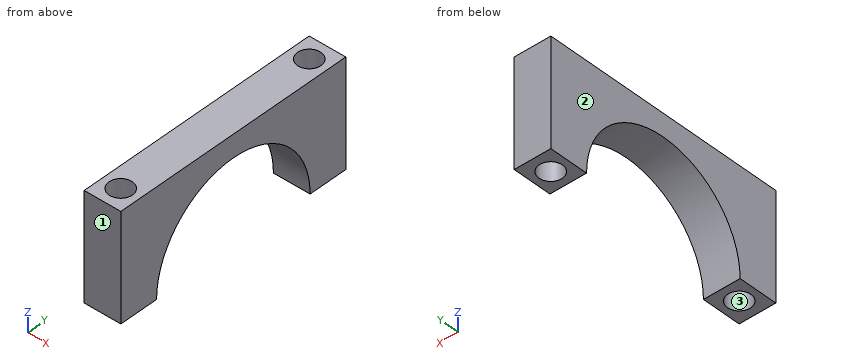
Autodesk Inventor part; units mm, degrees
ref_plane "YZ Plane" through (0, 0, 0) normal (1, 0, 0) x (0, 1, 0)
ref_plane "XZ Plane" through (0, 0, 0) normal (0, 1, 0) x (-1, 0, 0)
ref_plane "XY Plane" through (0, 0, 0) normal (0, 0, 1) x (1, 0, 0)
sketch "Sketch1" plane through (0, 0, 0) normal (0, 0, 1) x (1, 0, 0)
  line L0 (0, 0) -> (5.5, 0)
  line L1 (5.5, 0) -> (5.5, 37)
  line L2 (5.5, 37) -> (0, 37)
  line L3 (0, 37) -> (0, 0)
  point P0 (2.75, 34)
  point P1 (2.75, 3)
  dimension "d7" = 5.5
  dimension "d8" = 37
  dimension "d9" = 31
  dimension "d10" = 3
  dimension "d11" = 2.75
extrude "Extrusion4" add sketch "Sketch1" along normal blind 16
sketch "Sketch6" plane through (0, 0, 0) normal (0, 0, 1) x (1, 0, 0)
  line L0 (0, 0) -> (5.5, 0)
  line L1 (5.5, 0) -> (5.5, 37)
  line L2 (5.5, 37) -> (0, 37)
  line L3 (0, 37) -> (0, 0)
  point P0 (2.75, 34)
  point P1 (2.75, 3)
  dimension "d45" = 5.5
  dimension "d46" = 37
  dimension "d47" = 31
  dimension "d48" = 3
  dimension "d49" = 2.75
hole "Hole3" at (2.75, 34, 0) at (2.75, 3, 0) direction (0, 0, 1) diameter 3.5 end through all
sketch "Sketch7" plane through (5.5, 0, 0) normal (1, 0, 0) x (0, 0, -1)
  line L0 (0, 0) -> (0, 37)
  arc A0 (0, 31.125) -> (0, 5.875) centre (0, 18.5) ccw
  line L1 (0, 31.125) -> (0, 5.875)
  dimension "d59" = 25.25
extrude "Extrusion5" cut sketch "Sketch7" against normal blind 5.5
properties part number "SujetadorColaVTOL"
The listing builds one solid part. Answer for the finished solid, in the listing's coordinates (mm). Face numbers are marked on the shaded views. Give positions to 0.01 mm unless a question says otherwise; leave off trailing zeros. Order: outer loops, then holes, each group sorted by start corner. A loop starts at its lowest first (then second) coordinate and runs counter-clockwise, first axis right, second up. Notation, with made-up numbers: (15.5, 46.25) - (73.5, 46.25) arc R5 ccw to (73.5, 50.25) - close; hole circle Ø7 at (14, 68). An arc over 180 degrees is marked (long way). Answer as CSV lines item,"result".
Q1. A cutting plane is placed at D-D, the plane z = 2.25. Determine the outline of the cut face in (x, y), and give its area (3 significant figures).
Answer key:
outline,"(0, 0) - (5.5, 0) - (5.5, 6.08) - (0, 6.08) - close; (0, 30.92) - (5.5, 30.92) - (5.5, 37) - (0, 37) - close; hole circle Ø3.5 at (2.75, 3); hole circle Ø3.5 at (2.75, 34)"
area,"47.6 mm^2"
Q2. A cutting plane is placed at C-C, the plane x = 1.35. Determine the outline of the cut face in (y, z) (3 decimals).
Answer key:
outline,"(0, 0) - (1.95, 0) - (1.95, 16) - (0, 16) - close; (4.05, 0) - (5.875, 0) arc R12.625 cw to (31.125, 0) - (32.95, 0) - (32.95, 16) - (4.05, 16) - close; (35.05, 0) - (37, 0) - (37, 16) - (35.05, 16) - close"
Q3. A cutting plane is placed at B-B, the plane z = 4. Determine the outline of the cut face in (x, y).
Answer key:
outline,"(0, 0) - (5.5, 0) - (5.5, 6.53) - (0, 6.53) - close; (0, 30.47) - (5.5, 30.47) - (5.5, 37) - (0, 37) - close; hole circle Ø3.5 at (2.75, 3); hole circle Ø3.5 at (2.75, 34)"
Q4. Determine the mould class of the marked faces 1, 2 and 3 for opening direction Y: pulls with the +Y half, pulls with the -Y half, needs draft (parallel to the pull), parting line crosses it, or undercut.
Answer key:
face 1,"pulls with the -Y half"
face 2,"needs draft"
face 3,"undercut"
Q5. A cutting plane is placed at A-A, the plane y = 3. Determine the outline of the cut face in (x, z).
Answer key:
outline,"(0, 0) - (1, 0) - (1, 16) - (0, 16) - close; (4.5, 0) - (5.5, 0) - (5.5, 16) - (4.5, 16) - close"
Q6. Straight lines are drawn through the part: L1, parallel to Y at x = 2.75, z = 6; L2, parallel to Y at x = 4.3, z = 7.25; L3, parallel to X at y = 3, z = 4.75. For each, find the intervals that lie inside material, in ascending order.
Answer key:
L1,"y = 0 to 1.25, 4.75 to 7.39, 29.61 to 32.25, 35.75 to 37"
L2,"y = 0 to 2.19, 3.81 to 8.16, 28.84 to 33.19, 34.81 to 37"
L3,"x = 0 to 1, 4.5 to 5.5"
